Solid Edge part; units mm, degrees
sketch "Sketch1" plane through (0, 0, 0) normal (0, 0, 1) x (1, 0, 0)
  line L0 (-90.035, -90.095) -> (90.035, -90.095)
  line L1 (90.035, -90.095) -> (90.035, 90.095)
  line L2 (90.035, 90.095) -> (-90.035, 90.095)
  line L3 (-90.035, 90.095) -> (-90.035, -90.095)
  dimension "D1" = 90.035
  dimension "D2" = 90.035
extrude "Protrusion1" add sketch "Sketch1" along normal blind 3
sketch "Sketch2" plane through (0, 0, 3) normal (0, 0, 1) x (1, 0, 0)
  line L0 (-90.035, -70.095) -> (90.035, -70.095)
  line L1 (90.035, -70.095) -> (90.035, 70.095)
  line L2 (90.035, 70.095) -> (-90.035, 70.095)
  line L3 (-90.035, 70.095) -> (-90.035, -70.095)
extrude "Extrusionsausprägung_2" add sketch "Sketch2" along normal blind 3
sketch "Sketch3" plane through (0, -90, 3) normal (0, 0, 1) x (1, 0, 0)
  line L0 (-70, 9.905) -> (70, 9.905)
  line L1 (70, 9.905) -> (70, 19.905)
  line L2 (70, 19.905) -> (-70, 19.905)
  line L3 (-70, 19.905) -> (-70, 9.905)
  dimension "D1" = 70
extrude "Cutout1" cut sketch "Sketch3" against normal through all
mirror "Mirror1" about plane through (0, 0, 0) normal (0, -1, 0) of "Cutout1"
sketch "Sketch4" plane through (0, 0, 0) normal (0, 0, -1) x (-1, 0, 0)
  circle A0 centre (-30.035, -28.445) radius 3.5
  circle A1 centre (-30.035, 51.555) radius 3.5
  dimension "D1" = 30.035
  dimension "D2" = 30.035
extrude "Cutout3" cut sketch "Sketch4" against normal through all
properties material "Nylon, allgemein"
The model under review builds one solid part; all positions refer to its coordinate system, in mm. A direction names the side the tool comes from. Coordinates: 2 decimals unless noted, no trailing zeros. Write each loop counter-clockwise with the first axis right and the second up, starting at its lowest first coordinate (ties: lowest second). Pieces come first, ordered by that corner, then holes.
1) Machinability: for faces 5 (the face through (-1, 82, 3)), 6 (the face through (26.697, 52.606, 2.958)), 7 (the face through (-1, -84, 3)), which of the approach directions +Z, -Z, +X, -X, +Y, -Y give a long, thin tool a straight path to every point of the face, cutting with its end or side? Answer none if there is none.
2) The part is to be moulded in two halves that separate along X. For faces 1 (the face through (-1, 1, 6)), 2 (the face through (-1, -70.095, 3)), 3 (the face through (1, 70.095, 3)), 4 (the face through (-90.035, 1, 3)), say which applies: pulls with the +X half, pulls with the -X half, needs draft (parallel to the pull), parting line crosses it, or undercut.
3) We need section C-C on z = 1.75. State the section outline as (x, y) points (3 decimals).
4) We need section A-A on x = 47. State the section outline as (y, z) points (3 decimals).
5) To check wall thickness, follow probe 1 along Y at (x, z) = (60, 2.7) (3 decimals); probe 2 along Y at (x, z) = (30, 4.25) (3 decimals); probe 3 along Y at (x, z) = (8.5, 5.75) (3 decimals). State the ranges of each line that lie inside material, in increasing order.
6) We need section B-B on x = -74.5. State the section outline as (y, z) points (3 decimals), then the cut area to 3 significant figures.
7) Clearance check with flat-ended pins moving along their axes: pin 1 Ø12 at (x, y) = (-34.5, -55.5) entering from -Z; pin 2 Ø6 at (x, y) = (-34.5, -84.5) entering from +Z. State where each tip first meets the part, or that it passes through.
Answer list:
1. face 5: +Z, +X, -X, +Y
1. face 6: +Z, -Z
1. face 7: +Z, +X, -X, -Y
2. face 1: needs draft
2. face 2: undercut
2. face 3: undercut
2. face 4: pulls with the -X half
3. outline: (-90.035, -90.095) - (90.035, -90.095) - (90.035, 90.095) - (-90.035, 90.095) - close; hole (-70, -80.095) - (70, -80.095) - (70, -70.095) - (-70, -70.095) - close; hole (-70, 70.095) - (70, 70.095) - (70, 80.095) - (-70, 80.095) - close; hole circle Ø7 at (30.035, -28.445); hole circle Ø7 at (30.035, 51.555)
4. outline: (-90.095, 0) - (-80.095, 0) - (-80.095, 3) - (-90.095, 3) - close; (-70.095, 0) - (70.095, 0) - (70.095, 6) - (-70.095, 6) - close; (80.095, 0) - (90.095, 0) - (90.095, 3) - (80.095, 3) - close
5. probe 1: y = -90.095 to -80.095, -70.095 to 70.095, 80.095 to 90.095
5. probe 2: y = -70.095 to -31.945, -24.945 to 48.055, 55.055 to 70.095
5. probe 3: y = -70.095 to 70.095
6. outline: (-90.095, 0) - (90.095, 0) - (90.095, 3) - (70.095, 3) - (70.095, 6) - (-70.095, 6) - (-70.095, 3) - (-90.095, 3) - close
6. area: 961 mm2
7. pin 1: stops at z = 0
7. pin 2: stops at z = 3
